```python
from build123d import *

# Parameters (mm, degrees)
F1_DEPTH = 60
F3_DEPTH = 25
F5_DEPTH = 5.5
F7_DEPTH = 25
F9_DEPTH = 4
F11_D    = 2.5


with BuildPart() as f1:
    # F0 (on Front) → F1 (new body, symmetric)
    with BuildSketch(Plane.XZ):
        Polygon((-14.5, 2.2), (-14.5, 0), (14.5, 0), (14.5, 2.2), (17.0033320997, 2.2), (12.5, 10), (-12.5, 10), (-17.0033320997, 2.2), align=None)
    extrude(amount=F1_DEPTH, both=True)

    # F2 (on face) → F3 (cut)
    with BuildSketch(Plane.XY.offset(10)):
        with BuildLine():
            ThreePointArc((-4.5, 0), (-6.5, 2), (-8.5, 0))
            Line((-8.5, 0), (-8.5, -52))
            ThreePointArc((-8.5, -52), (-6.5, -54), (-4.5, -52))
            Line((-4.5, -52), (-4.5, 0))
        make_face()
        with BuildLine():
            ThreePointArc((8.5, 0), (6.5, 2), (4.5, 0))
            Line((4.5, 0), (4.5, -52))
            ThreePointArc((4.5, -52), (6.5, -54), (8.5, -52))
            Line((8.5, -52), (8.5, 0))
        make_face()
    extrude(amount=-F3_DEPTH, mode=Mode.SUBTRACT)

    # F4 (on face) → F5 (cut)
    with BuildSketch(Plane(origin=(0, 0, 0), x_dir=(1, 0, 0), z_dir=(0, 0, -1))):
        with BuildLine():
            ThreePointArc((-10.5, 0), (-6.5, -4), (-2.5, 0))
            Line((-2.5, 0), (-2.5, 52))
            ThreePointArc((-2.5, 52), (-6.5, 56), (-10.5, 52))
            Line((-10.5, 52), (-10.5, 0))
        make_face()
        with BuildLine():
            ThreePointArc((-4.5, 0), (-6.5, -2), (-8.5, 0))
            Line((-8.5, 0), (-8.5, 52))
            ThreePointArc((-8.5, 52), (-6.5, 54), (-4.5, 52))
            Line((-4.5, 52), (-4.5, 0))
        make_face(mode=Mode.SUBTRACT)
        with BuildLine():
            ThreePointArc((2.5, 0), (6.5, -4), (10.5, 0))
            Line((10.5, 0), (10.5, 52))
            ThreePointArc((10.5, 52), (6.5, 56), (2.5, 52))
            Line((2.5, 52), (2.5, 0))
        make_face()
        with BuildLine():
            ThreePointArc((4.5, 52), (6.5, 54), (8.5, 52))
            Line((8.5, 52), (8.5, 0))
            ThreePointArc((8.5, 0), (6.5, -2), (4.5, 0))
            Line((4.5, 0), (4.5, 52))
        make_face(mode=Mode.SUBTRACT)
    extrude(amount=-F5_DEPTH, mode=Mode.SUBTRACT)

    # F6 (on face) → F7 (cut)
    with BuildSketch(Plane(origin=(0, 0, 0), x_dir=(1, 0, 0), z_dir=(0, 0, -1))):
        with BuildLine():
            ThreePointArc((0, 60), (7.6113304895, 58.8131822355), (14.5, 55.3654118544))
            Line((14.5, 55.3654118544), (14.5, 60))
            Line((14.5, 60), (0, 60))
        make_face()
        with BuildLine():
            ThreePointArc((-14.5, 55.3654118544), (-7.6113304895, 58.8131822355), (0, 60))
            Line((0, 60), (-14.5, 60))
            Line((-14.5, 60), (-14.5, 55.3654118544))
        make_face()
        with BuildLine():
            ThreePointArc((14.5, 55.3654118544), (18.1961519016, 52.1435135248), (21.1923439056, 48.2621476311))
            Line((21.1923439056, 48.2621476311), (21.1923439056, 66.2593638897))
            Line((21.1923439056, 66.2593638897), (-20.7064654678, 66.2593638897))
            Line((-20.7064654678, 66.2593638897), (-20.7064654678, 49.0086504643))
            ThreePointArc((-20.7064654678, 49.0086504643), (-17.8878703743, 52.4649389771), (-14.5, 55.3654118544))
            Line((-14.5, 55.3654118544), (-14.5, 60))
            Line((-14.5, 60), (0, 60))
            Line((0, 60), (14.5, 60))
            Line((14.5, 60), (14.5, 55.3654118544))
        make_face()
    extrude(amount=-F7_DEPTH, mode=Mode.SUBTRACT)

    # F8 (on face) → F9 (cut)
    with BuildSketch(Plane.XY.offset(10)):
        Polygon((12.5, 60), (-12.5, 60), (-26.1883419007, 60), (-26.1883419007, 52), (21.1705399538, 52), (21.1705399538, 60), align=None)
    extrude(amount=-F9_DEPTH, mode=Mode.SUBTRACT)

    # F11 (through all)
    with Locations(Plane.XY.offset(6)):
        with Locations((9, 56), (-9, 56)):
            Hole(F11_D / 2)


solid = f1.part
```
The model under review builds one solid part; all positions refer to its coordinate system, in mm. A direction names the side the tool comes from. Round coordinates to 2 decimals unless told otherwise and drop trailing zeros. Loops run counter-clockwise (first coordinate to the right, second up) from the corner with the lowest first, then second, coordinate; pieces in that order, holes last.
1) The part is to be moulded in two halves that separate along X. For faces 6 (the face through (-14.72, 0.858, 6.155)), 7 (the face through (6.5, 2, 7.8)), 8 (the face through (16, 2, 2.2)), say which applies: pulls with the +X half, pulls with the -X half, needs draft (parallel to the pull), parting line crosses it, or undercut.
Values follow:
face 6: pulls with the -X half
face 7: undercut
face 8: needs draft
2) Consider section D-D on y = 19.5. State the section outline as (x, z) points.
Values follow:
outline: (-17, 2.2) - (-14.5, 2.2) - (-14.5, 0) - (14.5, 0) - (14.5, 2.2) - (17, 2.2) - (12.5, 10) - (-12.5, 10) - close
3) Consider section A-A on y = 56. State the section outline as (x, z) points.
Values follow:
outline: (-17, 2.2) - (-14.5, 2.2) - (-14.5, 0) - (-10.25, 0) - (-10.25, 6) - (-14.81, 6) - close; (-7.75, 0) - (7.75, 0) - (7.75, 6) - (-7.75, 6) - close; (10.25, 0) - (14.5, 0) - (14.5, 2.2) - (17, 2.2) - (14.81, 6) - (10.25, 6) - close
4) Consider section B-B on z = 8.25. State the section outline as (x, y) points.
Values follow:
outline: (-13.51, -56.03) arc R25 ccw to (13.51, -56.03) - (13.51, 52) - (-13.51, 52) - close; hole (-8.5, -52) arc R2 ccw to (-4.5, -52) - (-4.5, 0) arc R2 ccw to (-8.5, 0) - close; hole (4.5, -52) arc R2 ccw to (8.5, -52) - (8.5, 0) arc R2 ccw to (4.5, 0) - close
5) Consider section C-C on x = 6.5. State the section outline as (y, z) points, then the cut area to 3 significant figures.
Values follow:
outline: (-59.14, 0) - (-56, 0) - (-56, 5.5) - (-54, 5.5) - (-54, 10) - (-59.14, 10) - close; (2, 5.5) - (4, 5.5) - (4, 0) - (60, 0) - (60, 6) - (52, 6) - (52, 10) - (2, 10) - close
area: 577 mm2
6) Clearance check with flat-ended pins moving along their axes: P1, Ø6, axis at y = -20, z = 1.5, coming from the +X side; P2, Ø9, axis at x = -5.5, y = 55, coming from the +Z side; P3, Ø5, axis at x = -5.5, y = -4, coming from the -Z side; P4, Ø5, axis at y = 42.5, z = 5, coming from the +X side. State where each tip first meets the part, or that it passes through.
Values follow:
P1: stops at x = 17
P2: stops at z = 10
P3: stops at z = 5.5
P4: stops at x = 16.83
7) Tool access review of faces 1 (the face through (-6.5, -54, 7.8)), 2 (the face through (0, 52, 8)), 3 (the face through (-6.6, 4, 2.7)), 4 (the face through (0, -5, 10)), 5 (the face through (0, 12, 0)): name each direction out of +Z, -Z, +X, -X, +Y, -Y from which nothing blocks a thin tool from reaching the whole face with its end or side.
Values follow:
face 1: +Z, -Z
face 2: +Z, +X, -X, +Y
face 3: -Z
face 4: +Z, +X, -X, +Y, -Y
face 5: -Z, +X, -X, +Y, -Y
8) Wall thickness on line 1 along X through (y, z) = (-21, 6); line 2 along X through (y, z) = (-28, 6.25); line 3 along Y through (x, z) = (-9, 2.35): over which ranges is each line inside the solid? List them lowest first.
Values follow:
line 1: x = -14.81 to -8.5, -4.5 to 4.5, 8.5 to 14.81
line 2: x = -14.67 to -8.5, -4.5 to 4.5, 8.5 to 14.67
line 3: y = -58.32 to -55.12, 3.12 to 54.75, 57.25 to 60
